Source: CAD feature listing. Evaluate the final solid. Frame: model axes, mm. A direction names the side the tool comes from. Give positions to 0.01 mm unless a question says otherwise; leave off trailing zeros. Write each loop counter-clockwise with the first axis right and the second up, starting at its lowest first coordinate (ties: lowest second). Pieces come first, ordered by that corner, then holes. Notation, with made-up numbers: (-1.5, 83.5) -> (28.5, 83.5) arc R22 cw to (28.5, 94.5) -> close; hole circle Ø6 at (18.5, 82.5). An arc over 180 degrees is marked (long way). Answer as a JSON object with one key per item and string values. Group by question number.
Item 1: Section query B-B on y = -11.5. Give the number of separate pieces and of enclosed holes in the cut face, plus the area to 3 significant figures.
Item 2: Section query C-C on x = -976. Return the cut outline in (y, z), plus the area to 3 significant figures.
Item 3: Access query for faces 1 (the face through (-1043.016, -9.392, 113.658)), 2 (the face through (-1086.764, -9.658, 148.403)). Directions: +Z, -Z, +X, -X, +Y, -Y. A direction counts if a zero-diameter tool reaches every point of the face in a straight line with its end or side. Return the directions, or none.
Item 4: First-contact query: pin 1 Ø1 at (x, y) = (-636.5, -9.5) entering from +Z; pin 2 Ø10 at (x, y) = (-898.5, -6.5) entering from +Z; pin 3 Ø10 at (x, y) = (-929, -16) entering from +Z. Flat tips, straight axial feed; report the tip coordinate or a pass-through.
Item 5: Section query A-A on x = -387. Return the cut outline in (y, z), plus the area to 4 significant figures.
Item 6: Pull-direction query (Z, two-part tool) for faces 3 (the face through (-316.4, -9.39, 309.96)), 4 (the face through (-875, -10, 50)), 5 (the face through (-651.487, -9.658, 252.256)), 6 (the face through (-1081.96, -9.66, 17.11)); classes: pulls with the +Z half, pulls with the -Z half, needs draft (parallel to the pull), parting line crosses it, or undercut.
Item 7: Ray query, probe 1 along X at (y, z) = (-12.5, 113.5); probe 2 along Z at (x, y) = (-351.5, -1); probe 3 along X at (y, z) = (-15.5, 23). Return the intervals inside material, ascending. Write a range as from..to.
from build123d import *

# Parameters (mm, degrees)
F1_DEPTH = 19.05
F2_R     = 6.35
F3_DEPTH = 25
F4_R     = 6.35
F5_DEPTH = 25
F6_DEPTH = 25
F7_W     = 202.144652
F7_H     = 274.999976
F8_DEPTH = 25
F9_R     = 50
F10_R    = 60
F11_R    = 25
F12_R    = 30


with BuildPart() as f1:
    # F0 (on Front) → F1 (new body)
    with BuildSketch(Plane.XZ):
        Polygon((-1100, 0), (0, 0), (0, 375), (-525, 375), (-650, 250), (-1100, 160), align=None)
    extrude(amount=F1_DEPTH)

    # F2 (on face) → F3 (cut)
    with BuildSketch(Plane.XZ.offset(19.05)):
        with Locations((-325, 25)):
            Circle(F2_R)
    extrude(amount=-F3_DEPTH, mode=Mode.SUBTRACT)

    # F4 (on face) → F5 (cut)
    with BuildSketch(Plane.XZ.offset(19.05)):
        with Locations((-25, 25)):
            Circle(F4_R)
    extrude(amount=-F5_DEPTH, mode=Mode.SUBTRACT)

    # F4 (on face) → F6 (cut)
    with BuildSketch(Plane.XZ.offset(19.05)):
        with Locations((-25, 25)):
            Circle(F4_R)
    extrude(amount=F6_DEPTH, mode=Mode.SUBTRACT)

    # F7 (on face) → F8 (cut)
    with BuildSketch(Plane.XZ.offset(19.05)):
        Polygon((-675.34939, 50.000012), (-675.34939, 193.939915), (-1049.999988, 119.009795), (-1049.999988, 50.000012), align=None)
        Polygon((-504.289317, 324.999988), (-625.34939, 203.939915), (-625.34939, 50.000012), (-302.144664, 50.000012), (-302.144664, 324.999988), align=None)
        with Locations((-151.072338, 187.5)):
            Rectangle(F7_W, F7_H)
    extrude(amount=-F8_DEPTH, mode=Mode.SUBTRACT)

    # F9
    f9_edges = [f1.edges().sort_by_distance(p)[0] for p in [
        (-675.34939, -9.525, 50.000012),
        (-675.34939, -9.525, 193.939915),
        (-625.34939, -9.525, 203.939915),
        (-625.34939, -9.525, 50.000012),
        (-504.289317, -9.525, 324.999988),
        (-302.144664, -9.525, 324.999988),
        (-302.144664, -9.525, 50.000012),
        (-50.000012, -9.525, 50.000012),
        (-252.144664, -9.525, 50.000012),
        (-252.144664, -9.525, 324.999988),
        (-50.000012, -9.525, 324.999988),
    ]]
    fillet(f9_edges, radius=F9_R)

    # F10
    f10_edges = [f1.edges().sort_by_distance(p)[0] for p in [
        (-650, -9.525, 250),
        (-525, -9.525, 375),
        (0, -9.525, 375),
        (-1100, -9.525, 160),
        (-1100, -9.525, 0),
    ]]
    fillet(f10_edges, radius=F10_R)

    # F11
    f11_edges = [f1.edges().sort_by_distance(p)[0] for p in [
        (0, -9.525, 0),
    ]]
    fillet(f11_edges, radius=F11_R)

    # F12
    f12_edges = [f1.edges().sort_by_distance(p)[0] for p in [
        (-1049.999988, -9.525, 119.009795),
        (-1049.999988, -9.525, 50.000012),
    ]]
    fillet(f12_edges, radius=F12_R)


solid = f1.part
Worked answers:
{
 "1": {"separate pieces": "1", "enclosed holes": "5", "area": "154,000 mm^2"},
 "2": {"outline": "(-19.05, 0) -> (0, 0) -> (0, 50) -> (-19.05, 50) -> close; (-19.05, 133.81) -> (0, 133.81) -> (0, 184.8) -> (-19.05, 184.8) -> close", "area": "1,920 mm^2"},
 "3": {"face 1": "+Y, -Y", "face 2": "+Z, -X, +Y, -Y"},
 "4": {"pin 1": "z = 264", "pin 2": "z = 201.3", "pin 3": "z = 195.2"},
 "5": {"outline": "(-19.05, 0) -> (0, 0) -> (0, 50) -> (-19.05, 50) -> close; (-19.05, 325) -> (0, 325) -> (0, 375) -> (-19.05, 375) -> close", "area": "1,905 mm^2"},
 "6": {"face 3": "undercut", "face 4": "undercut", "face 5": "pulls with the +Z half", "face 6": "pulls with the -Z half"},
 "7": {"probe 1": "-1099.94..-1043.15, -675.35..-625.35, -302.14..-252.14, -50..0", "probe 2": "0..50, 325..375", "probe 3": "-1087.23..-331.03, -318.97..-31.03, -18.97..-0.08"}
}
